from build123d import *

# Parameters (mm, degrees)
F1_DEPTH = 6


with BuildPart() as f1:
    # F0 (on Top) → F1 (new body)
    with BuildSketch(Plane.XY):
        with BuildLine():
            ThreePointArc((-201.463409, 326.604773), (-194.963409, 333.104773), (-188.463409, 326.604773))
            Line((-188.463409, 326.604773), (-188.463409, 51.954773))
            ThreePointArc((-188.463409, 51.954773), (-186.559603, 47.358579), (-181.963409, 45.454773))
            Line((-181.963409, 45.454773), (157.736591, 45.453617))
            Line((157.736591, 45.453617), (157.736591, 46.754773))
            Line((157.736591, 46.754773), (-181.963409, 46.754773))
            ThreePointArc((-181.963409, 46.754773), (-185.640364, 48.277818), (-187.163409, 51.954773))
            Line((-187.163409, 51.954773), (-187.163409, 326.604773))
            ThreePointArc((-187.163409, 326.604773), (-194.963409, 334.404773), (-202.763409, 326.604773))
            Line((-202.763409, 326.604773), (-202.763409, -153.395227))
            ThreePointArc((-202.763409, -153.395227), (-200.478842, -158.910659), (-194.963409, -161.195227))
            Line((-194.963409, -161.195227), (262.736591, -161.195227))
            ThreePointArc((262.736591, -161.195227), (268.252024, -158.910659), (270.536591, -153.395227))
            Line((270.536591, -153.395227), (270.536591, 38.954837))
            ThreePointArc((270.536591, 38.954837), (268.263179, 44.459093), (262.768173, 46.754773))
            Line((262.768173, 46.754773), (232.736591, 46.754773))
            Line((232.736591, 46.754773), (232.736591, 45.453361))
            Line((232.736591, 45.453361), (262.879846, 45.453259))
            ThreePointArc((262.879846, 45.453259), (267.383157, 43.500101), (269.236591, 38.954837))
            Line((269.236591, 38.954837), (269.236591, -153.395227))
            ThreePointArc((269.236591, -153.395227), (267.332785, -157.991421), (262.736591, -159.895227))
            Line((262.736591, -159.895227), (-194.963409, -159.895227))
            ThreePointArc((-194.963409, -159.895227), (-199.559603, -157.991421), (-201.463409, -153.395227))
            Line((-201.463409, -153.395227), (-201.463409, 326.604773))
        make_face()
    extrude(amount=F1_DEPTH)


solid = f1.part
The listing builds one solid part. Answer for the finished solid, in the listing's coordinates (mm). Round coordinates to 2 decimals unless told otherwise and drop trailing zeros. Order: outer loops, then holes, each group sorted by start corner. A loop starts at its lowest first (then second) coordinate and runs counter-clockwise, first axis right, second up. Notation, with made-up numbers: (60, -25.75) -> (87, -25.75) arc R12 ccw to (87, -13.75) -> close; hole circle Ø10 at (10.5, -13). An arc over 180 degrees is marked (long way). Write each question's results on one line, items separated by ' | '. Start each with the question number.
Q1. Each of these flat-tipped pins is pushed along its axis until it touches: pin 1 (1 mm diameter, centred on y = 46.5, z = 4, fed in from +X); pin 2 (2 mm diameter, centred on x = -77, z = 1, fed in from +Y); pin 3 (1.8 mm diameter, centred on y = 247.5, z = 4.5, fed in from +X). Where does it stop, or does it pass through?
Q2. Find section A-A (y = 245.5). Determine the outline of the cut face in (x, z), then the cut area to 3 significant figures.
Q3. Find section B-B (x = 98). Determine the outline of the cut face in (y, z), then the cut area to 3 significant figures.
Q4. Find section C-C (z = 3.1). Determine the outline of the cut face in (x, y), then the cut area to 3 significant figures.
Q5. Straight lines are drawn through the part: probe 1 along X at (y, z) = (192, 3.7); probe 2 along X at (y, z) = (-73.5, 2.55); probe 3 along Y at (x, z) = (73, 5). For each, find the intervals that lie inside material, in ascending order. Write a range as from..to.
Worked answers:
1) pin 1: stops at x = 266.08 | pin 2: stops at y = 46.75 | pin 3: stops at x = -187.16
2) outline: (-202.76, 0) -> (-201.46, 0) -> (-201.46, 6) -> (-202.76, 6) -> close; (-188.46, 0) -> (-187.16, 0) -> (-187.16, 6) -> (-188.46, 6) -> close | area: 15.6 mm2
3) outline: (-161.2, 0) -> (-159.9, 0) -> (-159.9, 6) -> (-161.2, 6) -> close; (45.45, 0) -> (46.75, 0) -> (46.75, 6) -> (45.45, 6) -> close | area: 15.6 mm2
4) outline: (-202.76, -153.4) arc R7.8 ccw to (-194.96, -161.2) -> (262.74, -161.2) arc R7.8 ccw to (270.54, -153.4) -> (270.54, 38.95) arc R7.8 ccw to (262.77, 46.75) -> (232.74, 46.75) -> (232.74, 45.45) -> (262.88, 45.45) arc R6.5 cw to (269.24, 38.95) -> (269.24, -153.4) arc R6.5 cw to (262.74, -159.9) -> (-194.96, -159.9) arc R6.5 cw to (-201.46, -153.4) -> (-201.46, 326.6) arc R6.5 cw to (-188.46, 326.6) -> (-188.46, 51.95) arc R6.5 ccw to (-181.96, 45.45) -> (157.74, 45.45) -> (157.74, 46.75) -> (-181.96, 46.75) arc R5.2 cw to (-187.16, 51.95) -> (-187.16, 326.6) arc R7.8 ccw to (-202.76, 326.6) -> close | area: 2,390 mm2
5) probe 1: x = -202.76..-201.46, -188.46..-187.16 | probe 2: x = -202.76..-201.46, 269.24..270.54 | probe 3: y = -161.2..-159.9, 45.45..46.75
